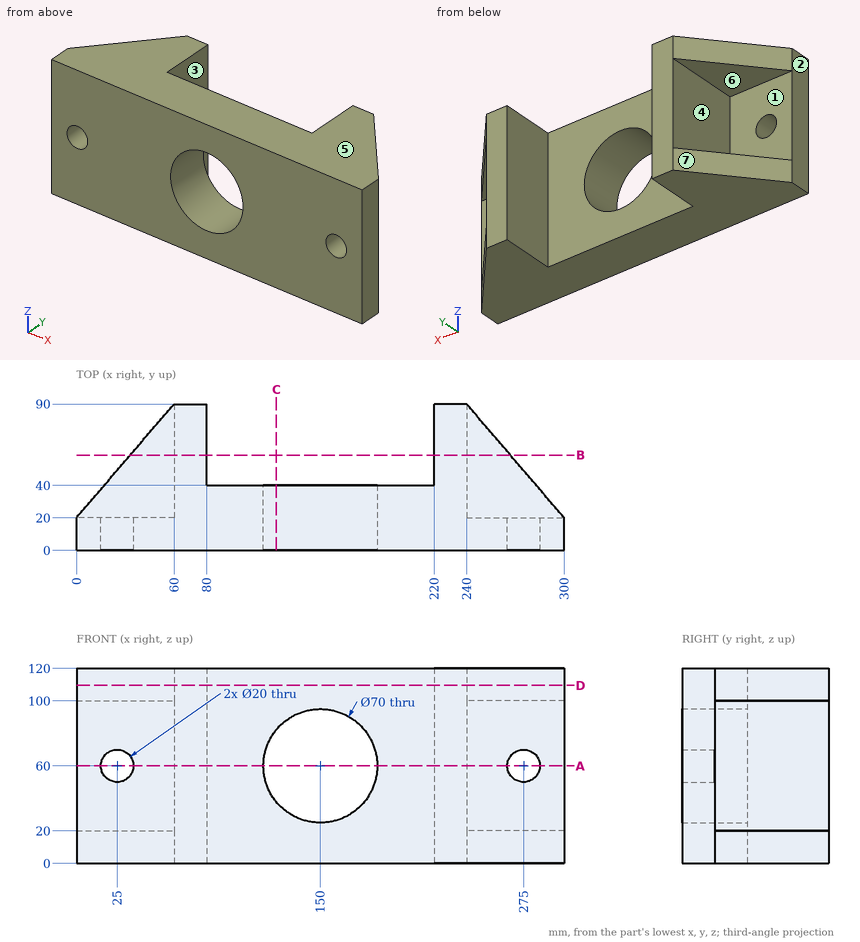
The figure shows three views and two pictorial views of one solid part (mm, origin at its lowest corner). Answer the questions. A direction names the side the tool comes from. Give positions to 0.01 mm unless a question says otherwise; leave off trailing zeros. Write each loop counter-clockwise with the first axis right and the second up, starting at its lowest first coordinate (ties: lowest second). Pieces come first, ordered by that corner, then holes. Notation, with made-up numbers: (-16.75, 29) - (10.25, 29) arc R10 ccw to (10.25, 45) - close; hole circle Ø8 at (5.25, 18.25). An arc over 180 degrees is marked (long way). Return JSON: item names as keys, results as strings.
Q1. Consider line 1 along X through (y, z) = (56, 42); line 2 along Z through (x, y) = (247, 49); line 3 along Z through (x, y) = (275, 7.25). Determine where each line is inside the solid, lowest interval first. Write a range as [from, to].
Reply:
{"line 1": "[60, 80], [220, 240]", "line 2": "[0, 20], [100, 120]", "line 3": "[0, 50], [70, 120]"}
Q2. For a pull along Z with two mould halves and no side action, classify the marked faces 4, 5, 6 and 7 as released by +Z, released by -Z, zero draft, split by the parting line, or undercut.
Reply:
{"face 4": "undercut", "face 5": "released by +Z", "face 6": "undercut", "face 7": "zero draft"}
Q3. For the marked faces 1, 2 and 3, determine the directions among +Z, -Z, +X, -X, +Y, -Y from which every point of the face is accessible in a straight line to the end or side of a thin tool.
Reply:
{"face 1": "-X, +Y", "face 2": "+Z, -Z, -X, +Y, -Y", "face 3": "+Z, -Z, +Y"}
Q4. A cutting plane is placed at A-A, the plane z = 60. Determine the outline of the cut face in (x, y).
Reply:
{"outline": "(0, 0) - (15, 0) - (15, 20) - (0, 20) - close; (35, 0) - (115, 0) - (115, 40) - (80, 40) - (80, 90) - (60, 90) - (60, 20) - (35, 20) - close; (185, 0) - (265, 0) - (265, 20) - (240, 20) - (240, 90) - (220, 90) - (220, 40) - (185, 40) - close; (285, 0) - (300, 0) - (300, 20) - (285, 20) - close"}
Q5. A cutting plane is placed at B-B, the plane y = 58.5. Determine the outline of the cut face in (x, z).
Reply:
{"outline": "(33, 0) - (80, 0) - (80, 120) - (33, 120) - (33, 100) - (60, 100) - (60, 20) - (33, 20) - close; (220, 0) - (267, 0) - (267, 20) - (240, 20) - (240, 100) - (267, 100) - (267, 120) - (220, 120) - close"}
Q6. A cutting plane is placed at C-C, the plane x = 123. Determine the outline of the cut face in (y, z), and give its area (3 significant figures).
Reply:
{"outline": "(0, 0) - (40, 0) - (40, 37.73) - (0, 37.73) - close; (0, 82.27) - (40, 82.27) - (40, 120) - (0, 120) - close", "area": "3,020 mm²"}
Q7. A cutting plane is placed at D-D, the plane z = 109.5. Determine the outline of the cut face in (x, y).
Reply:
{"outline": "(0, 0) - (300, 0) - (300, 20) - (240, 90) - (220, 90) - (220, 40) - (80, 40) - (80, 90) - (60, 90) - (0, 20) - close"}
Q8. Given P1, Ø2, axis at y = 77.5, z = 43.5, coming from the +X side; P2, Ø4, axis at x = 162.5, z = 105, coming from the +Y side; P3, Ø4, axis at y = 54, z = 88.5, coming from the -X side, each flat-ended and moving along its own axis, determine where each tip first touches the part or whether it passes through.
Reply:
{"P1": "x = 240", "P2": "y = 40", "P3": "x = 60"}
